Part model, mm, in its own coordinate system. Face numbers are marked on the shaded views. A direction names the side the tool comes from. Give positions to 0.01 mm unless a question says otherwise; leave off trailing zeros. Write each loop counter-clockwise with the first axis right and the second up, starting at its lowest first coordinate (ties: lowest second). Pieces come first, ordered by that corner, then holes. Notation, with made-up numbers: M -19,21.5 L 5,21.5 A36 ccw 5,57.5 Z; hole C 24,-9 d6. An arc over 180 degrees is marked long. Answer as CSV lines item,"result". Start each with the question number.
1) Pin check, flat tips, straight feed: pin 1 Ø1.5 at (x, z) = (3.5, 42) entering from -Y; pin 2 Ø6 at (x, y) = (-20, 115) entering from +Z; pin 3 Ø10 at (y, z) = (106.5, 12) entering from -X (3 decimals). Stop position of each tip, or through.
2) Slice it at A-A, the plane x = 20. Give the cut face in (y, z) (1 decimal), plus the area to 3 significant figures.
3) Wall check: line 1 along X through (y, z) = (96.5, 51) (3 decimals); line 2 along Z through (x, y) = (30.5, 84); line 3 along Y through (x, z) = (19.5, 53). Give the ranges that are in metal, low to high. Write a range as from..to.
4) Slice it at C-C, the plane y = 123. Give the cut face in (x, z) (3 decimals).
5) Tool access for the marked faces 1 and 2: list every direction of +Z, -Z, +X, -X, +Y, -Y with a clear straight run to the whole face (end or side of a thin tool).
6) Slice it at B-B, the plane z = 72. Give the cut face in (x, y) (3 decimals).
7) Slice it at D-D, the plane x = -1. Give the cut face in (y, z) (1 decimal), plus the area to 3 significant figures.
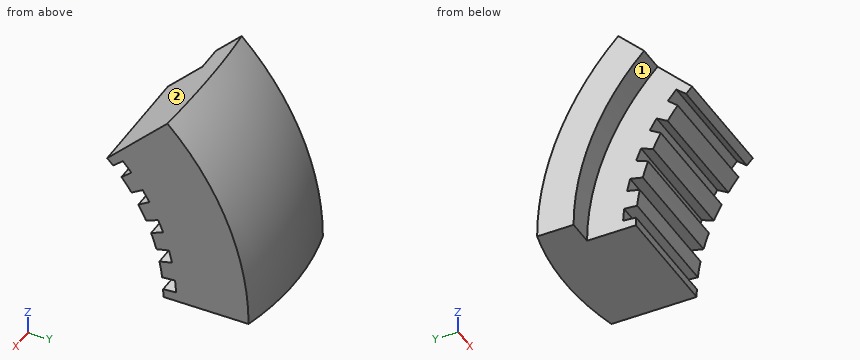
Autodesk Inventor part; units mm, degrees
ref_plane "Work Plane1" through (34.925, 0, 0) normal (0, 0, 1) x (0, 1, 0)
ref_plane "YZ Plane" through (0, 0, 0) normal (1, 0, 0) x (0, 1, 0)
ref_plane "XZ Plane" through (0, 0, 0) normal (0, 1, 0) x (-1, 0, 0)
sketch "Sketch1" plane through (0, 0, 0) normal (0, 0, 1) x (1, 0, 0)
  circle A0 centre (0, 0) radius 139.7
  line L0 (0, 139.7) -> (234.2216, 139.7) construction
  line L1 (-34.925, 185.7375) -> (34.925, 185.7375) construction
  line L2 (34.925, 185.7375) -> (34.925, 93.6625)
  line L3 (34.925, 93.6625) -> (-34.925, 93.6625)
  line L4 (-34.925, 93.6625) -> (-34.925, 185.7375)
  line L5 (-34.925, 185.7375) -> (34.925, 93.6625) construction
  line L6 (34.925, 185.7375) -> (-34.925, 93.6625) construction
  line L7 (0, 0) -> (253.8576, 0) construction
  point P0 (-34.925, 135.2639)
  point P1 (34.925, 135.2639)
  dimension "d6" = 279.4
  dimension "d7" = 69.85
  dimension "d8" = 92.075
  dimension "d9" = 93.6625
revolve "Revolution2" add sketch "Sketch1" angle 360 about axis through (0, 0, 0) along (1, 0, 0) picked at (2.3523, 108.9489) contours L2 L3 L4 A0
sketch "Sketch4" plane through (-34.925, 0, 0) normal (-1, 0, 0) x (0, 0, 1)
  circle A0 centre (0, 0) radius 93.6625
  circle A1 centre (0, 0) radius 117.475
  dimension "d24" = 234.95
extrude "Extrusion3" cut sketch "Sketch4" against normal blind 12.7
sketch "Sketch5" plane through (34.925, 0, 0) normal (1, 0, 0) x (0, 0, -1)
  circle A0 centre (0, 0) radius 93.6625
  circle A1 centre (0, 0) radius 135.2639
  line L0 (0, 0) -> (0, 180.6754)
  line L1 (0, 0) -> (-127.7568, 127.7568)
  line L2 (0, 0) -> (-180.6754, 0)
  line L3 (0, 0) -> (-127.7568, -127.7568)
  line L4 (0, 0) -> (0, -180.6754)
  line L5 (0, 0) -> (127.7568, -127.7568)
  line L6 (0, 0) -> (180.6754, 0)
  line L7 (0, 0) -> (127.7568, 127.7568)
  dimension "d29" = 360
ref_plane "Work Plane1" through (34.925, 0, 0) normal (0, 0, 1) x (0, 1, 0)
pattern_circular "Circular Pattern1" count 8 over 360 about axis through (0, 0, 0) along (1, 0, 0)
split "Split1" plane through (34.925, 0, 0) removes the side toward (0, 0, -1)
split "Split2" plane through (34.925, 0, 0) removes the side toward (0, -0.7071068, 0.7071068)
sketch "Sketch6" plane through (-22.225, 0, 0) normal (-1, 0, 0) x (0, 0, 1)
  arc A0 (66.2294, 66.2294) -> (0, 93.6625) centre (0, 0) ccw
  line L0 (0, 0) -> (75.2096, 181.5721) construction
  line L1 (0, 0) -> (196.5323, 0) construction
  line L2 (32.8892, 87.6982) -> (38.7558, 85.2681)
  line L3 (38.7558, 85.2681) -> (41.1858, 91.1348)
  line L4 (41.1858, 91.1348) -> (35.3192, 93.5648)
  line L5 (35.3192, 93.5648) -> (32.8892, 87.6982)
  line L6 (38.2525, 92.3498) -> (35.8225, 86.4831)
  dimension "d37" = 67.5
  dimension "d46" = 6.35
  dimension "d48" = 6.35
extrude "Extrusion4" cut sketch "Sketch6" against normal up to next
pattern_circular "Circular Pattern2" count 40 over 360 about axis through (0, 0, 0) along (1, 0, 0) of "Extrusion4" geometry pattern yes
ref_plane "Work Plane2" through (34.925, 0, 0) normal (0, -0.7071068, 0.7071068) x (0, 0.7071068, 0.7071068)
ref_plane "Work Plane3" through (34.925, 0, 0) normal (0, -1, 0) x (0, 0, 1)
ref_plane "Work Plane4" through (34.925, 0, 0) normal (0, -0.7071068, -0.7071068) x (0, -0.7071068, 0.7071068)
ref_plane "Work Plane5" through (34.925, 0, 0) normal (0, 0, -1) x (0, -1, 0)
ref_plane "Work Plane6" through (34.925, 0, 0) normal (0, 0.7071068, -0.7071068) x (0, -0.7071068, -0.7071068)
ref_plane "Work Plane7" through (34.925, 0, 0) normal (0, 1, 0) x (0, 0, -1)
ref_plane "Work Plane8" through (34.925, 0, 0) normal (0, 0.7071068, 0.7071068) x (0, 0.7071068, -0.7071068)
properties part number "bigWheelWedge01" material "Wood (Maple)"
Found:
1,pin 1,"y = 83.34"
1,pin 2,"z = 81.13"
1,pin 3,"x = -22.225"
2,outline,"M 66.2,66.2 A93.7 cw 69.1,63.2 L 73.9,67.3 L 78.1,62.5 L 73.2,58.4 A93.7 cw 78.2,51.6 L 83.6,54.9 L 86.9,49.5 L 81.5,46.2 A93.7 cw 85.3,38.8 L 91.1,41.2 L 93.6,35.3 L 87.7,32.9 A93.7 cw 90.3,24.9 L 96.5,26.4 L 97.9,20.2 L 91.8,18.8 A93.7 cw 93.1,10.5 L 99.4,11 L 99.9,4.7 L 93.6,4.2 A93.7 cw 93.7,0 L 138.3,0 A138.3 ccw 97.8,97.8 Z"
2,area,"3,860 mm²"
3,line 1,"-22.225..34.925"
3,line 2,"41.43..47.75, 54.23..84"
3,line 3,"77.22..80.41, 84.76..127.78"
4,outline,"M -34.925,0 L 34.925,0 L 34.925,56.279 A66.235 ccw -34.925,56.279 Z"
5,face 1,"-Z, -X, -Y"
5,face 2,"+Z, +X, -X, -Y"
6,outline,"M -34.925,92.824 L -22.225,92.824 L -22.225,72 L 34.925,72 L 34.925,114.509 A119.717 ccw -34.925,114.509 Z"
7,outline,"M 66.2,66.2 A93.7 cw 69.1,63.2 L 73.9,67.3 L 78.1,62.5 L 73.2,58.4 A93.7 cw 78.2,51.6 L 83.6,54.9 L 86.9,49.5 L 81.5,46.2 A93.7 cw 85.3,38.8 L 91.1,41.2 L 93.6,35.3 L 87.7,32.9 A93.7 cw 90.3,24.9 L 96.5,26.4 L 97.9,20.2 L 91.8,18.8 A93.7 cw 93.1,10.5 L 99.4,11 L 99.9,4.7 L 93.6,4.2 A93.7 cw 93.7,0 L 139.7,0 A139.7 ccw 98.8,98.8 Z"
7,area,"4,020 mm²"
